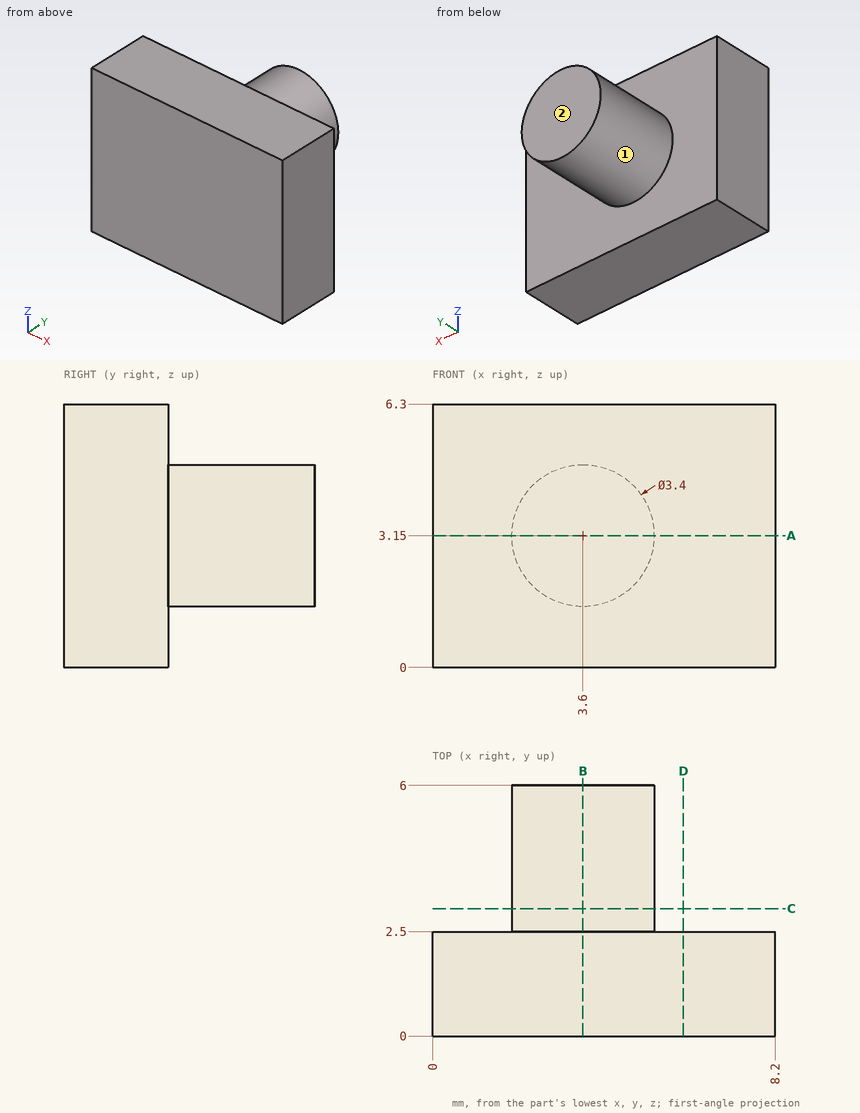
Answer from the drawing. Dimensions are ordinates in mm from the lowest x, y and z of the part. A direction names the side the tool comes from. Give positions to 0.01 mm unless a question says otherwise; leave off trailing zeros. Loops run counter-clockwise (first coordinate to the right, second up) from the corner with the lowest first, then second, coordinate; pieces in that order, holes last.
Item 1: Find the intervals of material crossed by line 1 along Y through (x, z) = (6, 1.5); line 2 along Z through (x, y) = (3.25, 4.8); line 3 along X through (y, z) = (5.7, 4.25), in increasing order.
Derived:
line 1: y = 0 to 2.5
line 2: z = 1.49 to 4.81
line 3: x = 2.3 to 4.9
Item 2: A cutting plane is placed at A-A (z = 3.15). Give the vertices of the cut face in (x, y), then the cut area to 3 significant figures.
Derived:
outline: (0, 0) - (8.2, 0) - (8.2, 2.5) - (5.3, 2.5) - (5.3, 6) - (1.9, 6) - (1.9, 2.5) - (0, 2.5) - close
area: 32.4 mm2
Item 3: A tool of negligible diameter and unlimited length cuts with its end or side. For the marked faces 1 and 2, from which of +Z, -Z, +X, -X, +Y, -Y can it reach the whole face along a straight path? Write none if from no direction.
Derived:
face 1: +Y
face 2: +Z, -Z, +X, -X, +Y
Item 4: A cutting plane is placed at B-B (x = 3.6). Give the vertices of the cut face in (y, z).
Derived:
outline: (0, 0) - (2.5, 0) - (2.5, 1.45) - (6, 1.45) - (6, 4.85) - (2.5, 4.85) - (2.5, 6.3) - (0, 6.3) - close
Item 5: This flat-tipped pin is pushed along its axis until it touches: pin 1 Ø3 at (y, z) = (5, 1) entering from +X. Where does it stop, or does it pass through?
Derived:
pin 1: stops at x = 5.17
Item 6: A cutting plane is placed at C-C (y = 3.05). Give the vertices of the cut face in (x, z).
Derived:
outline: circle Ø3.4 at (3.6, 3.15)
Item 7: A cutting plane is placed at D-D (x = 6). Give the vertices of the cut face in (y, z), then the cut area to 4 significant figures.
Derived:
outline: (0, 0) - (2.5, 0) - (2.5, 6.3) - (0, 6.3) - close
area: 15.75 mm2
